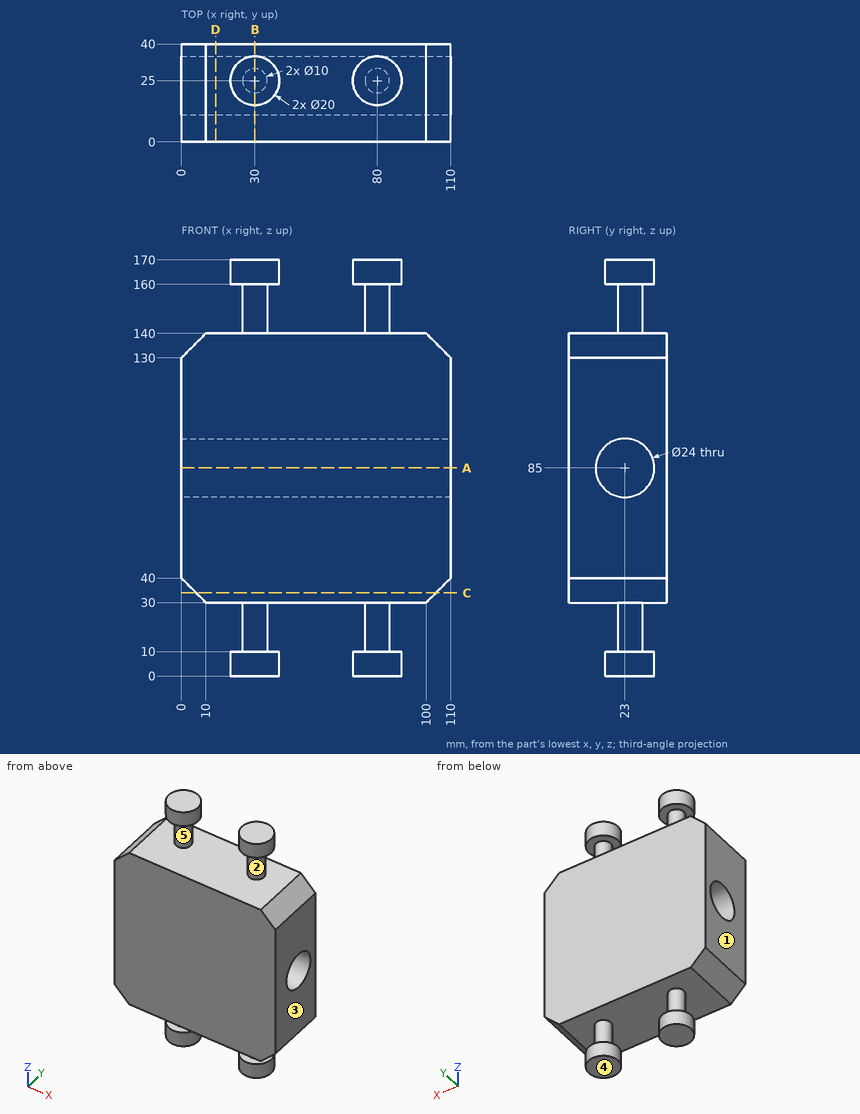
Geometry: see drawing. Coordinates: mm, zero at the bounding-box minimum. A direction names the side the tool comes from. Round coordinates to 2 decimals unless told otherwise and drop trailing zeros. Loops run counter-clockwise (first coordinate to the right, second up) from the corner with the lowest first, then second, coordinate; pieces in that order, holes last. Notation, with made-up numbers: M -37.5,31 L -11.5,31 A22 ccw -11.5,59 Z; hole C -22,86.5 d3. An arc over 180 degrees is marked long. Use a Markdown table: item, result. Add a question column.
1. Pull-direction query (X, two-part tool) for the marked faces 1, 2 and 3; classes: +X half, -X half, draft (parallel to the pull), parting line (faces both ways), or undercut.
2. Cut plane A-A, the plane z = 85. Output: boundary loops of the cut face in (x, y).
3. Cut plane C-C, the plane z = 34. Output: boundary loops of the cut face in (x, y), and give its area (3 significant figures).
4. Ray query, line 1 along Y through (x, z) = (45, 85); line 2 along Z through (x, y) = (81.5, 21.5); line 3 along Z through (x, y) = (34, 34). Return the intervals inside material, ascending. Write a range as [from, to].
5. Cut plane D-D, the plane x = 14. Output: boundary loops of the cut face in (y, z), and give its area (3 significant figures).
6. Set-up query: the marked faces 4 and 5. Return all of +Z, -Z, +X, -X, +Y, -Y with unobstructed straight access to the full face (end or side cutting, diameter ignored); none if empty.
7. Cut plane B-B, the plane x = 30. Output: boundary loops of the cut face in (y, z).
8. Contact query for flat-ended pins moving along their axis: pin 1 (12 mm diameter, centred on x = 52.5, y = 18, fed in from +Z); pin 2 (6 mm diameter, centred on x = 46, y = 7.5, fed in from -Z); pin 3 (4 mm diameter, centred on y = 11, z = 135, fed in from +X). Output: stop coordinate, or through.
Solution:
| question | item | result |
|---|---|---|
| 1 | face 1 | -X half |
| 1 | face 2 | undercut |
| 1 | face 3 | +X half |
| 2 | outline | M 0,0 L 110,0 L 110,11 L 0,11 Z; M 0,35 L 110,35 L 110,40 L 0,40 Z |
| 3 | outline | M 6,0 L 104,0 L 104,40 L 6,40 Z |
| 3 | area | 3,920 mm2 |
| 4 | line 1 | y = [0, 11], [35, 40] |
| 4 | line 2 | z = [0, 73.09], [96.91, 170] |
| 4 | line 3 | z = [0, 10], [30, 80.2], [89.8, 140], [160, 170] |
| 5 | outline | M 0,30 L 40,30 L 40,140 L 0,140 Z; hole C 23,85 d24 |
| 5 | area | 3,950 mm2 |
| 6 | face 4 | -Z, +X, -X, +Y, -Y |
| 6 | face 5 | none |
| 7 | outline | M 0,30 L 20,30 L 20,10 L 15,10 L 15,0 L 35,0 L 35,10 L 30,10 L 30,30 L 40,30 L 40,140 L 30,140 L 30,160 L 35,160 L 35,170 L 15,170 L 15,160 L 20,160 L 20,140 L 0,140 Z; hole C 23,85 d24 |
| 8 | pin 1 | stops at z = 140 |
| 8 | pin 2 | stops at z = 30 |
| 8 | pin 3 | stops at x = 107 |
